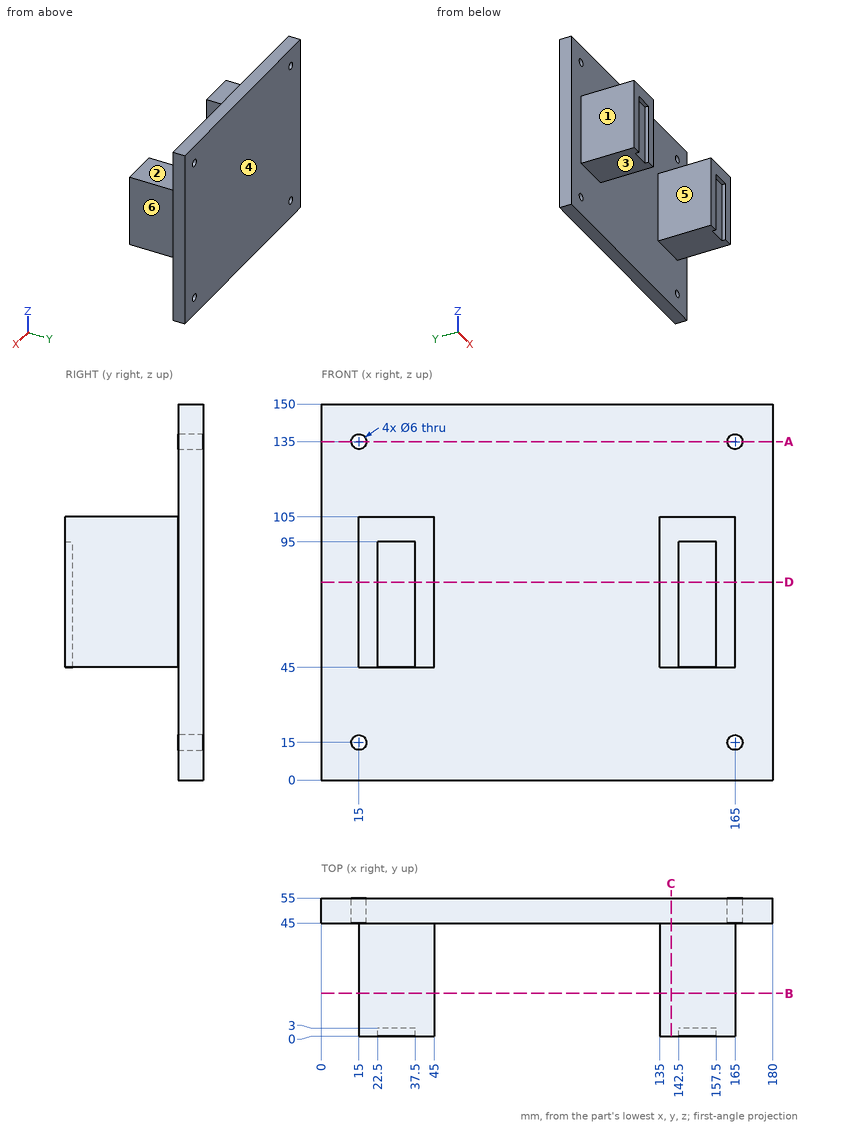
Source: three-view drawing plus pictorial views. Frame: mm from the lowest corner of the part. A direction names the side the tool comes from. Round coordinates to 2 decimals unless told otherwise and drop trailing zeros. Loops run counter-clockwise (first coordinate to the right, second up) from the corner with the lowest first, then second, coordinate; pieces in that order, holes last.
Q1. Mould query, pull axis X, two halves, no side actions, for the marked faces 4, 5 and 6. Classes: pulls with the +X half, pulls with the -X half, needs draft (parallel to the pull), parting line crosses it, or undercut.
Q2. First-contact query: P1, Ø16.5, axis at x = 148, z = 64, coming from the -Y side; P2, Ø10, axis at y = 9.5, z = 38.5, coming from the -X side; P3, Ø24, axis at x = 150.5, y = 30.5, coming from the +Z side; P4, Ø7.5, axis at x = 31, z = 62, coming from the -Y side. Flat tips, straight axial feed; report the tip coordinate or a pass-through.
Q3. Ray query, line 1 (Z direction, x = 165, y = 49); line 2 (X direction, y = 48, z = 15); line 3 (X direction, y = 27.5, z = 61.5). Return the intervals inside material, ascending.
Q4. Section D-D, the plane z = 79. Return loops of the section in (x, y).
Q5. Section C-C, the plane x = 139.5. Return loops of the section in (y, z).
Q6. Access query for the marked faces 1, 2 and 3. Directions: +Z, -Z, +X, -X, +Y, -Y. A direction counts if a zero-diameter tool reaches every point of the face in a straight line with its end or side. Return the directions, or none.
Q7. Section B-B, the plane y = 17. Return loops of the section in (x, z), plus the area to 3 significant figures.
Q8. Section A-A, the plane z = 135. Return loops of the section in (x, y).
Solutions:
1. face 4: needs draft
1. face 5: undercut
1. face 6: pulls with the +X half
2. P1: stops at y = 0
2. P2: passes through
2. P3: stops at z = 105
2. P4: stops at y = 3
3. line 1: z = 0 to 12, 18 to 132, 138 to 150
3. line 2: x = 0 to 12, 18 to 162, 168 to 180
3. line 3: x = 15 to 45, 135 to 165
4. outline: (0, 45) - (15, 45) - (15, 0) - (22.5, 0) - (22.5, 3) - (37.5, 3) - (37.5, 0) - (45, 0) - (45, 45) - (135, 45) - (135, 0) - (142.5, 0) - (142.5, 3) - (157.5, 3) - (157.5, 0) - (165, 0) - (165, 45) - (180, 45) - (180, 55) - (0, 55) - close
5. outline: (0, 45) - (45, 45) - (45, 0) - (55, 0) - (55, 150) - (45, 150) - (45, 105) - (0, 105) - close
6. face 1: +Z, -Z, -X, -Y
6. face 2: +Z, +X, -X, -Y
6. face 3: -Z, +X, -X, -Y
7. outline: (15, 45) - (45, 45) - (45, 105) - (15, 105) - close; (135, 45) - (165, 45) - (165, 105) - (135, 105) - close
7. area: 3,600 mm2
8. outline: (0, 45) - (12, 45) - (12, 55) - (0, 55) - close; (18, 45) - (162, 45) - (162, 55) - (18, 55) - close; (168, 45) - (180, 45) - (180, 55) - (168, 55) - close
